The listing builds one solid part. Answer for the finished solid, in the listing's coordinates (mm). A direction names the side the tool comes from. Give positions to 0.01 mm unless a question says otherwise; leave off trailing zeros. Write each loop counter-clockwise with the first axis right and the second up, starting at its lowest first coordinate (ties: lowest second). Pieces come first, ordered by that corner, then holes.
```python
from build123d import *

# Parameters (mm, degrees)
F1_DEPTH = 500
F2_DEPTH = 90


# Not quite as in the source:
# - a pattern or mirror of a feature is missing from the dataset's text; its kind, count and spacing are read off the source's solid


with BuildPart() as f1:
    # F0 (on Front) → F1 (new body)
    with BuildSketch(Plane.XZ):
        with BuildLine():
            Line((102, 0), (100, 0))
            Line((100, 0), (100, -11))
            ThreePointArc((100, -11), (99.4142135624, -12.4142135624), (98, -13))
            Line((98, -13), (0, -13))
            Line((0, -13), (-98, -13))
            ThreePointArc((-98, -13), (-99.4142135624, -12.4142135624), (-100, -11))
            Line((-100, -11), (-100, 0))
            Line((-100, 0), (-102, 0))
            Line((-102, 0), (-102, -13))
            ThreePointArc((-102, -13), (-101.4142135624, -14.4142135624), (-100, -15))
            Line((-100, -15), (100, -15))
            ThreePointArc((100, -15), (101.4142135624, -14.4142135624), (102, -13))
            Line((102, -13), (102, 0))
        make_face()
        with BuildLine():
            Line((105, 0), (102, 0))
            Line((102, 0), (102, -13))
            ThreePointArc((102, -13), (101.4142135624, -14.4142135624), (100, -15))
            Line((100, -15), (-100, -15))
            ThreePointArc((-100, -15), (-101.4142135624, -14.4142135624), (-102, -13))
            Line((-102, -13), (-102, 0))
            Line((-102, 0), (-105, 0))
            Line((-105, 0), (-105, -16))
            ThreePointArc((-105, -16), (-104.4142135624, -17.4142135624), (-103, -18))
            Line((-103, -18), (0, -18))
            Line((0, -18), (103, -18))
            ThreePointArc((103, -18), (104.4142135624, -17.4142135624), (105, -16))
            Line((105, -16), (105, 0))
        make_face()
    extrude(amount=F1_DEPTH)

    # F0 (on Front) → F2 (cut)
    with BuildSketch(Plane.XZ):
        with BuildLine():
            Line((105, 0), (102, 0))
            Line((102, 0), (102, -13))
            ThreePointArc((102, -13), (101.4142135624, -14.4142135624), (100, -15))
            Line((100, -15), (-100, -15))
            ThreePointArc((-100, -15), (-101.4142135624, -14.4142135624), (-102, -13))
            Line((-102, -13), (-102, 0))
            Line((-102, 0), (-105, 0))
            Line((-105, 0), (-105, -16))
            ThreePointArc((-105, -16), (-104.4142135624, -17.4142135624), (-103, -18))
            Line((-103, -18), (0, -18))
            Line((0, -18), (103, -18))
            ThreePointArc((103, -18), (104.4142135624, -17.4142135624), (105, -16))
            Line((105, -16), (105, 0))
        make_face()
    f2 = extrude(amount=F2_DEPTH, mode=Mode.SUBTRACT)

    # F2_copies: F2 across plane
    add(f2.mirror(Plane(origin=(0, -250, 0), x_dir=(0, 0, -1), z_dir=(0, -1, 0))), mode=Mode.SUBTRACT)


solid = f1.part
```
Item 1: A cutting plane is placed at C-C, the plane x = 65.5. Give the vertices of the cut face in (y, z), plus the area to 3 significant figures.
Conclusion:
outline: (-500, -15) - (-410, -15) - (-410, -18) - (-90, -18) - (-90, -15) - (0, -15) - (0, -13) - (-500, -13) - close
area: 1,960 mm2
Item 2: A cutting plane is placed at B-B, the plane y = -426. Give the vertices of the cut face in (x, z).
Conclusion:
outline: (-102, -13) arc R2 ccw to (-100, -15) - (100, -15) arc R2 ccw to (102, -13) - (102, 0) - (100, 0) - (100, -11) arc R2 cw to (98, -13) - (-98, -13) arc R2 cw to (-100, -11) - (-100, 0) - (-102, 0) - close
Item 3: A cutting plane is placed at A-A, the plane z = -5.75. Give the vertices of the cut face in (x, y).
Conclusion:
outline: (-105, -410) - (-102, -410) - (-102, -500) - (-100, -500) - (-100, 0) - (-102, 0) - (-102, -90) - (-105, -90) - close; (100, -500) - (102, -500) - (102, -410) - (105, -410) - (105, -90) - (102, -90) - (102, 0) - (100, 0) - close
Item 4: Determine the mould class of faces 6 (the face through (100, -246, -5)), 7 (the face through (0, -500, -14)), 8 (the face through (-102, -456, -7)) for opening direction X: pulls with the +X half, pulls with the -X half, needs draft (parallel to the pull), parting line crosses it, or undercut.
Conclusion:
face 6: undercut
face 7: needs draft
face 8: pulls with the -X half
Item 5: A cutting plane is placed at D-D, the plane y = -341.5. Give the vertices of the cut face in (x, z).
Conclusion:
outline: (-105, -16) arc R2 ccw to (-103, -18) - (103, -18) arc R2 ccw to (105, -16) - (105, 0) - (100, 0) - (100, -11) arc R2 cw to (98, -13) - (-98, -13) arc R2 cw to (-100, -11) - (-100, 0) - (-105, 0) - close
Item 6: Consider probe 1 along X at (y, z) = (-263, -6.5); probe 2 along Z at (x, y) = (28, -305); probe 3 along Y at (x, z) = (-85.5, -15.5). Determine where each line is inside the solid, lowest interval first.
Conclusion:
probe 1: x = -105 to -100, 100 to 105
probe 2: z = -18 to -13
probe 3: y = -410 to -90
Item 7: Which of the six approach directions +Z, -Z, +X, -X, +Y, -Y give full straight-line access (tool end or side, diameter ignored) to faces 1 (the face through (-100, -246, -6)), 2 (the face through (1, -44, -15)), 3 (the face through (1, -456, -15)), 4 (the face through (102, -456, -6)), 5 (the face through (102, -44, -6))?
Conclusion:
face 1: +Z, +Y, -Y
face 2: -Z, +X, -X, +Y
face 3: -Z, +X, -X, -Y
face 4: +Z, -Z, +X, -Y
face 5: +Z, -Z, +X, +Y
Item 8: Each of these flat-tipped pins is pushed along its axis until it touches: P1, Ø3, axis at x = -37.5, y = -257, coming from the +Z side; P2, Ø10.5, axis at y = -455.5, z = -8.5, coming from the +X side. Where does it stop, or does it pass through?
Conclusion:
P1: stops at z = -13
P2: stops at x = 102
